Can you work these out from the model? Positions are in its coordinate system, mm. A direction names the side the tool comes from. Give positions to 0.01 mm unless a question says otherwise; leave off trailing zeros. Order: outer loops, then holes, each group sorted by start corner. A loop starts at its lowest first (then second) coordinate and runs counter-clockwise, first axis right, second up.
```python
from build123d import *

# Parameters (mm, degrees)
SKETCH1_R           = 2.5
BOSS_EXTRUDE1_DEPTH = 150
FILLET1_R           = 1
FILLET2_R           = 0.5
FILLET3_R           = 0.5
FILLET4_R           = 0.5
FILLET5_R           = 0.5


with BuildPart() as part:
    # Sketch1 → Boss-Extrude1 (new body)
    with BuildSketch(Plane.XY):
        Polygon((13.2, 0), (13.2, 1.8), (15.45, 1.8), (15.45, 3.6), (12.95, 6.1), (7.05, 6.1), (4.55, 3.6), (4.55, 1.8), (6.8, 1.8), (6.8, 0), (0, 0), (0, 6.8), (1.8, 6.8), (1.8, 4.55), (3.6, 4.55), (6.1, 7.05), (6.1, 12.95), (3.6, 15.45), (1.8, 15.45), (1.8, 13.2), (0, 13.2), (0, 20), (6.8, 20), (6.8, 18.2), (4.55, 18.2), (4.55, 16.4), (7.05, 13.9), (12.95, 13.9), (15.45, 16.4), (15.45, 18.2), (13.2, 18.2), (13.2, 20), (20, 20), (20, 13.2), (18.2, 13.2), (18.2, 15.45), (16.4, 15.45), (13.9, 12.95), (13.9, 7.05), (16.4, 4.55), (18.2, 4.55), (18.2, 6.8), (20, 6.8), (20, 0), align=None)
        with Locations((10, 10)):
            Circle(SKETCH1_R, mode=Mode.SUBTRACT)
    extrude(amount=BOSS_EXTRUDE1_DEPTH)

    # Fillet1
    fillet1_edges = [part.edges().sort_by_distance(p)[0] for p in [
        (0, 0, 75),
        (0, 20, 75),
        (20, 20, 75),
        (20, 0, 75),
    ]]
    fillet(fillet1_edges, radius=FILLET1_R)

    # Fillet2
    fillet2_edges = [part.edges().sort_by_distance(p)[0] for p in [
        (4.55, 18.2, 75),
        (4.55, 16.4, 75),
        (7.05, 13.9, 75),
        (12.95, 13.9, 75),
        (15.45, 16.4, 75),
        (15.45, 18.2, 75),
    ]]
    fillet(fillet2_edges, radius=FILLET2_R)

    # Fillet3
    fillet3_edges = [part.edges().sort_by_distance(p)[0] for p in [
        (18.2, 15.45, 75),
        (16.4, 15.45, 75),
        (13.9, 12.95, 75),
        (13.9, 7.05, 75),
        (16.4, 4.55, 75),
        (18.2, 4.55, 75),
    ]]
    fillet(fillet3_edges, radius=FILLET3_R)

    # Fillet4
    fillet4_edges = [part.edges().sort_by_distance(p)[0] for p in [
        (1.8, 4.55, 75),
        (3.6, 4.55, 75),
        (6.1, 7.05, 75),
        (6.1, 12.95, 75),
        (3.6, 15.45, 75),
        (1.8, 15.45, 75),
    ]]
    fillet(fillet4_edges, radius=FILLET4_R)

    # Fillet5
    fillet5_edges = [part.edges().sort_by_distance(p)[0] for p in [
        (15.45, 1.8, 75),
        (15.45, 3.6, 75),
        (12.95, 6.1, 75),
        (7.05, 6.1, 75),
        (4.55, 3.6, 75),
        (4.55, 1.8, 75),
    ]]
    fillet(fillet5_edges, radius=FILLET5_R)


solid = part.part
```
1) Suppose I cut it at A-A (x = 10). Please give me the cut outline in (y, z).
2) I'm going to push flat-ended pins straight in: pin 1 Ø6 at (x, z) = (10, 81) entering from +Y; pin 2 Ø4.5 at (x, y) = (10, 10) entering from +Z; pin 3 Ø1.6 at (y, z) = (9, 78) entering from +X; pin 4 Ø4 at (x, z) = (10, 88) entering from +Y. Where does each tip first touch, or does it pass through?
3) We'd pull the mould along Y, two halves only. Please class faces 6 (the face through (16, 0, 74)), 7 (the face through (0, 16, 74)), 8 (the face through (13.9, 10, 74)): +Y half, -Y half, draft (parallel to the pull), parting line (faces both ways), or undercut.
4) If I drill on line 1 (Y direction, x = 10, z = 50.5); line 2 (Y direction, x = 3.75, z = 80); line 3 (X direction, y = 5.5, z = 38.5), over which ranges is the centre line in solid material (lowest first)?
5) Which directions (+Z, -Z, +X, -X, +Y, -Y) give clear straight access to the entire face, cutting with the end or side of a thin tool? Please do faces 1 (the face through (10, 13.9, 74)), 2 (the face through (6.1, 10, 74)), 3 (the face through (4, 0, 74)), 4 (the face through (10, 6.1, 74)), 5 (the face through (20, 16, 74)).
Results:
1. outline: (6.1, 0) - (7.5, 0) - (7.5, 150) - (6.1, 150) - close; (12.5, 0) - (13.9, 0) - (13.9, 150) - (12.5, 150) - close
2. pin 1: stops at y = 13.97
2. pin 2: passes through
2. pin 3: stops at x = 13.9
2. pin 4: stops at y = 13.9
3. face 6: -Y half
3. face 7: draft
3. face 8: undercut
4. line 1: y = 6.1 to 7.5, 12.5 to 13.9
4. line 2: y = 0 to 4.7, 15.3 to 20
4. line 3: x = 0 to 1.8, 4.55 to 6.45, 13.55 to 15.45, 18.2 to 20
5. face 1: +Z, -Z, +Y
5. face 2: +Z, -Z, -X
5. face 3: +Z, -Z, +X, -X, -Y
5. face 4: +Z, -Z, -Y
5. face 5: +Z, -Z, +X, +Y, -Y
